```python
from build123d import *

# Parameters (mm, degrees)
SKETCH_R         = 2.1
PAD_DEPTH        = 100
CHAMFER_1_ANGLE  = 45
CHAMFER_1_SIZE   = 1.7
CHAMFER_2_ANGLE  = 45
CHAMFER_2_SIZE   = 1.7
CHAMFER_3_ANGLE  = 45
CHAMFER_3_SIZE   = 1.7
CHAMFER_4_ANGLE  = 45
CHAMFER_4_SIZE   = 1.7
CHAMFER_5_ANGLE  = 45
CHAMFER_5_SIZE   = 1.7
CHAMFER_6_ANGLE  = 45
CHAMFER_6_SIZE   = 1.7
CHAMFER_7_ANGLE  = 45
CHAMFER_7_SIZE   = 1.7
CHAMFER_8_ANGLE  = 45
CHAMFER_8_SIZE   = 1.7
CHAMFER_9_ANGLE  = 45
CHAMFER_9_SIZE   = 1.7
CHAMFER_10_ANGLE = 45
CHAMFER_10_SIZE  = 1.7
CHAMFER_11_ANGLE = 45
CHAMFER_11_SIZE  = 1.7
CHAMFER_12_ANGLE = 45
CHAMFER_12_SIZE  = 1.7
FILLET_R         = 0.2


with BuildPart() as part:
    # Sketch → Pad (new body)
    with BuildSketch(Plane.XY):
        Polygon((0, 3.723883), (0.176777, 3.90066), (2.84, 3.90066), (5.49934, 6.56), (5.49934, 8.2), (3.1, 8.2), (3.1, 10), (16.9, 10), (16.9, 8.2), (14.50066, 8.2), (14.50066, 6.56), (17.16, 3.90066), (19.823223, 3.90066), (20, 3.723883), (20.176777, 3.90066), (22.84, 3.90066), (25.49934, 6.56), (25.49934, 8.2), (23.1, 8.2), (23.1, 10), (30, 10), (30, 3.1), (28.2, 3.1), (28.2, 5.49934), (26.56, 5.49934), (23.90066, 2.84), (23.90066, 0.176777), (23.723883, 0), (23.90066, -0.176777), (23.90066, -2.84), (26.56, -5.49934), (28.2, -5.49934), (28.2, -3.1), (30, -3.1), (30, -10), (23.1, -10), (23.1, -8.2), (25.49934, -8.2), (25.49934, -6.56), (22.84, -3.90066), (20.176777, -3.90066), (20, -3.723883), (19.823223, -3.90066), (17.16, -3.90066), (14.50066, -6.56), (14.50066, -8.2), (16.9, -8.2), (16.9, -10), (3.1, -10), (3.1, -8.2), (5.49934, -8.2), (5.49934, -6.56), (2.84, -3.90066), (0.176777, -3.90066), (0, -3.723883), (-0.176777, -3.90066), (-2.84, -3.90066), (-5.49934, -6.56), (-5.49934, -8.2), (-3.1, -8.2), (-3.1, -10), (-10, -10), (-10, -3.1), (-8.2, -3.1), (-8.2, -5.49934), (-6.56, -5.49934), (-3.90066, -2.84), (-3.90066, -0.176777), (-3.723883, 0), (-3.90066, 0.176777), (-3.90066, 2.84), (-6.56, 5.49934), (-8.2, 5.49934), (-8.2, 3.1), (-10, 3.1), (-10, 10), (-3.1, 10), (-3.1, 8.2), (-5.49934, 8.2), (-5.49934, 6.56), (-2.84, 3.90066), (-0.176777, 3.90066), align=None)
        Circle(SKETCH_R, mode=Mode.SUBTRACT)
        with Locations((20, 0)):
            Circle(SKETCH_R, mode=Mode.SUBTRACT)
        Polygon((7.29934, 6.23868), (3.90066, 2.84), (3.90066, 0.176777), (3.723883, 0), (3.90066, -0.176777), (3.90066, -2.84), (7.29934, -6.23868), (7.29934, -8.2), (12.70066, -8.2), (12.70066, -6.23868), (16.09934, -2.84), (16.09934, -0.176777), (16.276117, 0), (16.09934, 0.176777), (16.09934, 2.84), (12.70066, 6.23868), (12.70066, 8.2), (7.29934, 8.2), align=None, mode=Mode.SUBTRACT)
    extrude(amount=PAD_DEPTH)

    # Chamfer 1
    chamfer_1_edges = [part.edges().sort_by_distance(p)[0] for p in [
        (3.1, -10, 50),
    ]]
    chamfer_1_side = part.faces().sort_by_distance((10, -10, 50))[0]
    chamfer(chamfer_1_edges, length=CHAMFER_1_SIZE, angle=CHAMFER_1_ANGLE, reference=chamfer_1_side)

    # Chamfer 2
    chamfer_2_edges = [part.edges().sort_by_distance(p)[0] for p in [
        (16.9, -10, 50),
    ]]
    chamfer_2_side = part.faces().sort_by_distance((16.9, -9.1, 50))[0]
    chamfer(chamfer_2_edges, length=CHAMFER_2_SIZE, angle=CHAMFER_2_ANGLE, reference=chamfer_2_side)

    # Chamfer 3
    chamfer_3_edges = [part.edges().sort_by_distance(p)[0] for p in [
        (23.1, -10, 50),
    ]]
    chamfer_3_side = part.faces().sort_by_distance((26.55, -10, 50))[0]
    chamfer(chamfer_3_edges, length=CHAMFER_3_SIZE, angle=CHAMFER_3_ANGLE, reference=chamfer_3_side)

    # Chamfer 4
    chamfer_4_edges = [part.edges().sort_by_distance(p)[0] for p in [
        (-3.1, -10, 50),
    ]]
    chamfer_4_side = part.faces().sort_by_distance((-3.1, -9.1, 50))[0]
    chamfer(chamfer_4_edges, length=CHAMFER_4_SIZE, angle=CHAMFER_4_ANGLE, reference=chamfer_4_side)

    # Chamfer 5
    chamfer_5_edges = [part.edges().sort_by_distance(p)[0] for p in [
        (30, -3.1, 50),
    ]]
    chamfer_5_side = part.faces().sort_by_distance((29.1, -3.1, 50))[0]
    chamfer(chamfer_5_edges, length=CHAMFER_5_SIZE, angle=CHAMFER_5_ANGLE, reference=chamfer_5_side)

    # Chamfer 6
    chamfer_6_edges = [part.edges().sort_by_distance(p)[0] for p in [
        (30, 3.1, 50),
    ]]
    chamfer_6_side = part.faces().sort_by_distance((30, 6.55, 50))[0]
    chamfer(chamfer_6_edges, length=CHAMFER_6_SIZE, angle=CHAMFER_6_ANGLE, reference=chamfer_6_side)

    # Chamfer 7
    chamfer_7_edges = [part.edges().sort_by_distance(p)[0] for p in [
        (23.1, 10, 50),
    ]]
    chamfer_7_side = part.faces().sort_by_distance((23.1, 9.1, 50))[0]
    chamfer(chamfer_7_edges, length=CHAMFER_7_SIZE, angle=CHAMFER_7_ANGLE, reference=chamfer_7_side)

    # Chamfer 8
    chamfer_8_edges = [part.edges().sort_by_distance(p)[0] for p in [
        (16.9, 10, 50),
    ]]
    chamfer_8_side = part.faces().sort_by_distance((10, 10, 50))[0]
    chamfer(chamfer_8_edges, length=CHAMFER_8_SIZE, angle=CHAMFER_8_ANGLE, reference=chamfer_8_side)

    # Chamfer 9
    chamfer_9_edges = [part.edges().sort_by_distance(p)[0] for p in [
        (3.1, 10, 50),
    ]]
    chamfer_9_side = part.faces().sort_by_distance((3.1, 9.1, 50))[0]
    chamfer(chamfer_9_edges, length=CHAMFER_9_SIZE, angle=CHAMFER_9_ANGLE, reference=chamfer_9_side)

    # Chamfer 10
    chamfer_10_edges = [part.edges().sort_by_distance(p)[0] for p in [
        (-3.1, 10, 50),
    ]]
    chamfer_10_side = part.faces().sort_by_distance((-6.55, 10, 50))[0]
    chamfer(chamfer_10_edges, length=CHAMFER_10_SIZE, angle=CHAMFER_10_ANGLE, reference=chamfer_10_side)

    # Chamfer 11
    chamfer_11_edges = [part.edges().sort_by_distance(p)[0] for p in [
        (-10, -3.1, 50),
    ]]
    chamfer_11_side = part.faces().sort_by_distance((-10, -6.55, 50))[0]
    chamfer(chamfer_11_edges, length=CHAMFER_11_SIZE, angle=CHAMFER_11_ANGLE, reference=chamfer_11_side)

    # Chamfer 12
    chamfer_12_edges = [part.edges().sort_by_distance(p)[0] for p in [
        (-10, 3.1, 50),
    ]]
    chamfer_12_side = part.faces().sort_by_distance((-9.1, 3.1, 50))[0]
    chamfer(chamfer_12_edges, length=CHAMFER_12_SIZE, angle=CHAMFER_12_ANGLE, reference=chamfer_12_side)

    # Fillet
    fillet_edges = [part.edges().sort_by_distance(p)[0] for p in [
        (-10, -10, 50),
        (-10, 10, 50),
        (30, 10, 50),
        (30, -10, 50),
    ]]
    fillet(fillet_edges, radius=FILLET_R)


solid = part.part
```
Check sheet for the modelled part. Datum: model origin and axes. Units: mm. A direction names the side the tool comes from. Round coordinates to 2 decimals unless told otherwise and drop trailing zeros. Use CSV: the item, a comma, the result in double quotes.
(1) Cross-section at A-A (z = 50.5). Count the separate pieces of the cut face and the enclosed holes in it, and give its area (3 significant figures).
Worked out:
separate pieces,"1"
enclosed holes,"3"
area,"296 mm²"
(2) Draft check along Y on faces 5 (the face through (10, -10, 49)), 6 (the face through (10, 10, 49)), 7 (the face through (-3.901, 1, 49)). Enter one of: pulls with the +Y half, pulls with the -Y half, needs draft (parallel to the pull), parting line crosses it, or undercut.
Worked out:
face 5,"pulls with the -Y half"
face 6,"pulls with the +Y half"
face 7,"undercut"
(3) Tool access check on faces 1 (the face through (12.701, -7, 49)), 2 (the face through (16, -9.2, 49.3)), 3 (the face through (-2, 3.901, 49)), 4 (the face through (-10, -7, 49)). Record the directions out of +Z, -Z, +X, -X, +Y, -Y that give a thin tool (end or side, any length) a straight path to the whole face; none if there is none.
Worked out:
face 1,"+Z, -Z"
face 2,"+Z, -Z, -Y"
face 3,"+Z, -Z, +Y"
face 4,"+Z, -Z, -X, +Y, -Y"
(4) Material ranges on line 1 along X through (y, z) = (-7.25, 46); line 2 along Y through (x, z) = (0, 78.5); line 3 along X through (y, z) = (-4, 69), recorded low to high. Write a range as from..to.
Worked out:
line 1,"-10..-5.5, 5.5..7.3, 12.7..14.5, 25.5..30"
line 2,"-3.72..-2.1, 2.1..3.72"
line 3,"-9.2..-8.2, -5.06..-2.94, 2.94..5.06, 14.94..17.06, 22.94..25.06, 28.2..29.2"
(5) Depth check by flat-ended pin: pin 1 (0.8 mm diameter, centred on y = 2, z = 28.5, fed in from +X); pin 2 (5 mm diameter, centred on x = 24, y = -5, fed in from -Z); pin 3 (3 mm diameter, centred on x = 0.5, y = 0, fed in from +Z); pin 4 (1.3 mm diameter, centred on x = 1, z = 72, fed in from -Y). Enter the tip coordinate at first touch or a pass-through.
Worked out:
pin 1,"x = 23.9"
pin 2,"z = 0"
pin 3,"through"
pin 4,"y = -3.9"
